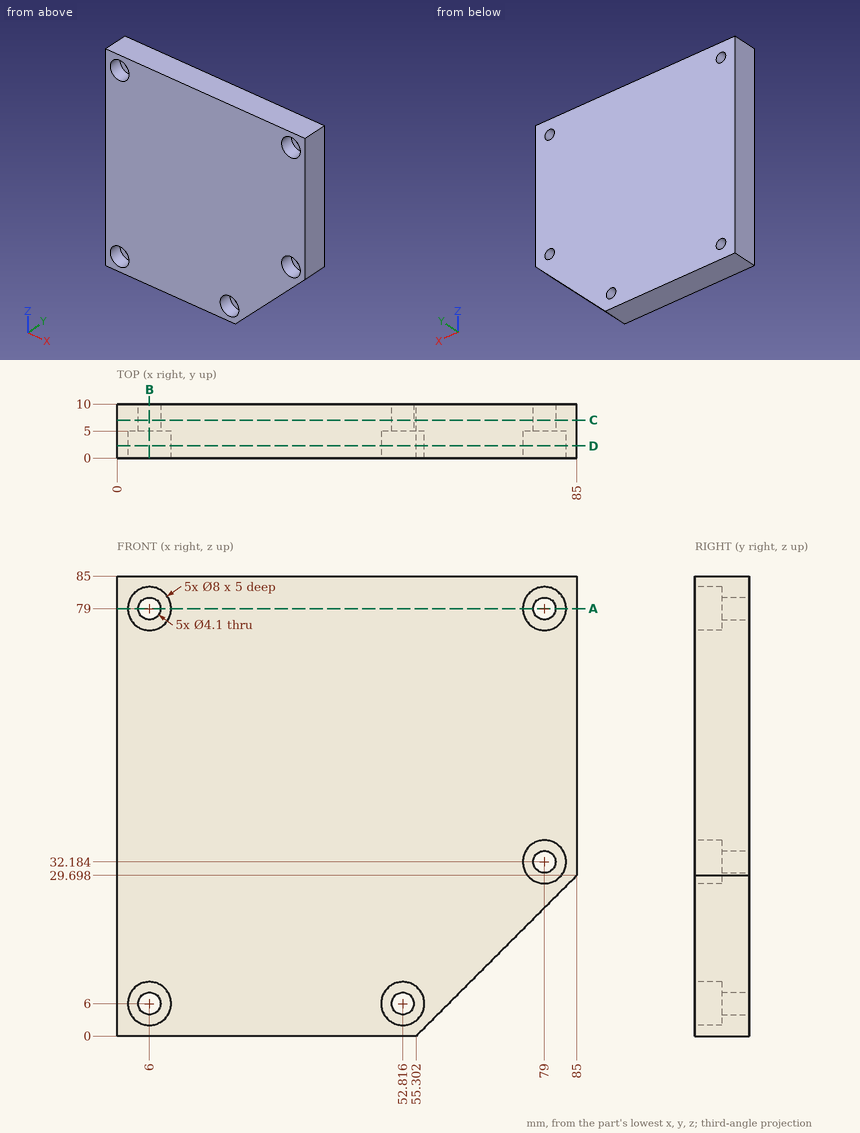
The figure shows three views and two pictorial views of one solid part (mm, origin at its lowest corner). Answer the questions. Give positions to 0.01 mm unless a question says otherwise; leave off trailing zeros. Loops run counter-clockwise (first coordinate to the right, second up) from the corner with the lowest first, then second, coordinate; pieces in that order, holes last. Notation, with made-up numbers: (86.5, 17.25) -> (103.5, 17.25) arc R4 ccw to (103.5, 24.25) -> close; hole circle Ø5 at (81.5, 26). An arc over 180 degrees is marked (long way). Use a Markdown table: item, result. Add a question column.
1. Section D-D on y = 2.25 is taken. Determine the outline of the cut face in (x, z).
2. Section A-A on z = 79 is taken. Determine the outline of the cut face in (x, y), and give its area (3 significant figures).
3. Section C-C on y = 7 is taken. Determine the outline of the cut face in (x, z).
4. Find the intervals of material crossed by probe 1 along Z at (x, y) = (6, 9.5); probe 2 along Z at (x, y) = (6, 3), in increasing order.
5. Section B-B on x = 6 is taken. Determine the outline of the cut face in (y, z), and give its area (3 significant figures).
6. A flat-ended cylindrical pin translates along its axis: pin 1 Ø6.5 at (x, z) = (79, 32.18) entering from -Y. Find the tip coordinate at first contact, or state that the pin passes through.
Results below:
| question | item | result |
|---|---|---|
| 1 | outline | (0, 0) -> (55.3, 0) -> (85, 29.7) -> (85, 85) -> (0, 85) -> close; hole circle Ø8 at (6, 6); hole circle Ø8 at (6, 79); hole circle Ø8 at (52.82, 6); hole circle Ø8 at (79, 32.18); hole circle Ø8 at (79, 79) |
| 2 | outline | (0, 0) -> (2, 0) -> (2, 5) -> (3.95, 5) -> (3.95, 10) -> (0, 10) -> close; (8.05, 5) -> (10, 5) -> (10, 0) -> (75, 0) -> (75, 5) -> (76.95, 5) -> (76.95, 10) -> (8.05, 10) -> close; (81.05, 5) -> (83, 5) -> (83, 0) -> (85, 0) -> (85, 10) -> (81.05, 10) -> close |
| 2 | area | 729 mm^2 |
| 3 | outline | (0, 0) -> (55.3, 0) -> (85, 29.7) -> (85, 85) -> (0, 85) -> close; hole circle Ø4.1 at (6, 6); hole circle Ø4.1 at (6, 79); hole circle Ø4.1 at (52.82, 6); hole circle Ø4.1 at (79, 32.18); hole circle Ø4.1 at (79, 79) |
| 4 | probe 1 | z = 0 to 3.95, 8.05 to 76.95, 81.05 to 85 |
| 4 | probe 2 | z = 0 to 2, 10 to 75, 83 to 85 |
| 5 | outline | (0, 0) -> (10, 0) -> (10, 3.95) -> (5, 3.95) -> (5, 2) -> (0, 2) -> close; (0, 10) -> (5, 10) -> (5, 8.05) -> (10, 8.05) -> (10, 76.95) -> (5, 76.95) -> (5, 75) -> (0, 75) -> close; (0, 83) -> (5, 83) -> (5, 81.05) -> (10, 81.05) -> (10, 85) -> (0, 85) -> close |
| 5 | area | 729 mm^2 |
| 6 | pin 1 | stops at y = 5 |
